Autodesk Inventor part; units mm, degrees
ref_plane "Work Plane1" through (50, 0, 0) normal (1, 0, 0) x (0, 1, 0)
ref_plane "XZ Plane" through (0, 0, 0) normal (0, 1, 0) x (-1, 0, 0)
ref_plane "XY Plane" through (0, 0, 0) normal (0, 0, 1) x (1, 0, 0)
sketch "Sketch1" plane through (0, 0, 0) normal (0, 1, 0) x (-1, 0, 0)
  circle A0 centre (0, 0) radius 50
  dimension "d0" = 100
extrude "Extrusion1" add sketch "Sketch1" along normal blind 20
ref_plane "Work Plane1" through (50, 0, 0) normal (1, 0, 0) x (0, 1, 0)
sketch "Sketch2" plane through (50, 0, 0) normal (1, 0, 0) x (0, 1, 0)
  line L0 (20, -50) -> (20, 50)
  line L1 (0, -50) -> (0, 50)
  point P0 (0, 0)
  point P1 (10, 0)
  dimension "d3" = 20
  dimension "d4" = 10
hole "Hole1" at (50, 10, 0) direction (-1, 0, 0) diameter 10 end through all
pattern_circular "Circular Pattern2" count 8 over 360 about axis through (0, -10, 0) along (0, 1, 0) of "Hole1"
sketch "Sketch4" plane through (0, 0, 0) normal (0, -1, 0) x (1, 0, 0)
  circle A0 centre (0, 0) radius 1
  dimension "d26" = 2
extrude "Extrusion2" cut sketch "Sketch4" against normal through all
sketch "Sketch5" plane through (0, 0, 0) normal (0, -1, 0) x (1, 0, 0)
  circle A0 centre (0, 0) radius 1
  line L0 (-11.4805, 27.7164) -> (0, 0)
  line L1 (0, 0) -> (0, 50)
  circle A1 centre (0, 0) radius 50
  point P0 (-27.7164, 11.4805)
  point P1 (-27.7164, -11.4805)
  point P2 (-11.4805, -27.7164)
  point P3 (11.4805, -27.7164)
  point P4 (27.7164, -11.4805)
  point P5 (27.7164, 11.4805)
  point P6 (11.4805, 27.7164)
  dimension "d31" = 30
  dimension "d32" = 22.5
  dimension "d35" = 360
hole "Hole3" at (-11.4805, 0, 27.7164) at (-27.7164, 0, 11.4805) at (-27.7164, 0, -11.4805) at (-11.4805, 0, -27.7164) at (11.4805, 0, -27.7164) at (27.7164, 0, -11.4805) at (27.7164, 0, 11.4805) at (11.4805, 0, 27.7164) direction (0, 1, 0) diameter 5 end through all
chamfer "Chamfer2" distance 1 angle 45 32 edges at (-49.8543, 6.7667, -3.8139) (-49.8545, 13.2353, -3.8122) (-49.8543, 13.2328, 3.8143) (-49.8544, 6.7652, 3.8126) (49.8545, 13.2353, -3.8122) (49.8543, 13.2328, 3.8143) (49.8543, 6.7667, -3.8139) (49.8544, 6.7652, 3.8126) (-37.9567, 6.7803, 32.5468) (-37.9554, 13.222, 32.5482) (-32.5468, 6.7803, 37.9567) (-32.5468, 13.2197, 37.9567) (32.5482, 13.222, -37.9554) (37.9567, 13.2197, -32.5468) (32.5468, 6.7803, -37.9567) (37.9567, 6.7803, -32.5468) (32.5468, 6.7803, 37.9567) (32.5482, 13.222, 37.9554) (37.9567, 6.7803, 32.5468) (37.9567, 13.2197, 32.5468) (-37.9554, 13.222, -32.5482) (-32.5468, 13.2197, -37.9567) (-37.9567, 6.7803, -32.5468) (-32.5468, 6.7803, -37.9567) (-3.8254, 6.7803, 49.8535) (-3.8235, 13.222, 49.8536) (3.8254, 6.7803, 49.8535) (3.8254, 13.2197, 49.8535) (-3.8235, 13.222, -49.8536) (3.8254, 13.2197, -49.8535) (-3.8254, 6.7803, -49.8535) (3.8254, 6.7803, -49.8535)
sketch "Sketch6" plane through (0, 20, 0) normal (0, 1, 0) x (1, 0, 0)
  circle A0 centre (0, 0) radius 60
  dimension "d50" = 120
extrude "Extrusion3" cut sketch "Sketch6" against normal blind 10.25
sketch "Sketch7" plane through (0, 9.75, 0) normal (0, 1, 0) x (1, 0, 0)
  circle A0 centre (0, 0) radius 17.5
  dimension "d53" = 35
extrude "Extrusion4" cut sketch "Sketch7" against normal blind 5
sketch "Sketch8" plane through (0, 0, 0) normal (0, -1, 0) x (1, 0, 0)
  point P0 (0, 0)
  point P1 (15.25, 0)
  point P2 (10.7834, 10.7834)
  point P3 (0, 15.25)
  point P4 (-10.7834, 10.7834)
  point P5 (-15.25, 0)
  point P6 (-10.7834, -10.7834)
  point P7 (0, -15.25)
  point P8 (10.7834, -10.7834)
  dimension "d56" = 15.25
  dimension "d59" = 360
hole "Hole4" at (15.25, 0, 0) at (10.7834, 0, 10.7834) at (0, 0, 15.25) at (-10.7834, 0, 10.7834) at (-15.25, 0, 0) at (-10.7834, 0, -10.7834) at (0, 0, -15.25) at (10.7834, 0, -10.7834) direction (0, 1, 0) diameter 2 end through all
sketch "Sketch9" plane through (0, 9.75, 0) normal (0, 1, 0) x (1, 0, 0)
  circle A0 centre (0, 0) radius 1
  circle A1 centre (0, 0) radius 60
  dimension "d68" = 120
extrude "Extrusion5" cut sketch "Sketch9" against normal blind 8.15
properties part number "CUT_FR4_Top_Disc_PCB"
Verification items for the finished model (mm, model axes). Round coordinates to 2 decimals unless told otherwise and drop trailing zeros. Order: outer loops, then holes, each group sorted by start corner. A loop starts at its lowest first (then second) coordinate and runs counter-clockwise, first axis right, second up. Notation, with made-up numbers: (57, 57.5) - (107, 57.5) arc R21 cw to (107, 76.5) - close; hole circle Ø2 at (-3, 61). An arc over 180 degrees is marked (long way). Use CSV: the item, a comma, the result in double quotes. Start each with the question number.
1) Go/stop test with a flat-tipped pin: P1, Ø4.5, axis at x = 11.48, z = -27.72, coming from the -Y side. Record where the tip stops, or that it passes through.
2) Thickness scan on L1, parallel to Z at x = 0, y = 0.6; L2, parallel to X at y = 0.25, z = 12.5. Record the ranges inside material, lowest first.
3) Mould release check, pull along X, two halves, no side actions. Record for faces 1 (the cylindrical face through (-25.276, 0.811, -10.939)), 2 (the cylindrical face through (-47.69, 0.79, -15.02)), 3 (the flat face through (1, 0, -10)): +X half, -X half, draft (parallel to the pull), parting line (faces both ways), or undercut.
4) Section check A-A, the plane y = 0.95. State how many separate pieces and enclosed holes the cut face has, plus the area to 3 significant figures.
5) Section check B-B, the plane x = -34. Record the cut outline in (y, z).
6) Section check C-C, the plane z = -33. Record the cut outline in (x, y).
Answers:
1,P1,"passes through"
2,L1,"z = -50 to -16.25, -14.25 to -1, 1 to 14.25, 16.25 to 50"
2,L2,"x = -48.41 to -30, -25.43 to 25.43, 30 to 48.41"
3,face 1,"undercut"
3,face 2,"parting line"
3,face 3,"draft"
4,separate pieces,"1"
4,enclosed holes,"17"
4,area,"7,670 mm²"
5,outline,"(0, -36.66) - (1.6, -36.66) - (1.6, 36.66) - (0, 36.66) - close"
6,outline,"(-37.56, 0) - (37.56, 0) - (37.56, 1.6) - (-37.56, 1.6) - close"
